```python
from build123d import *

# Parameters (mm, degrees)
SKETCH1_W                                 = 25.4
SKETCH1_H                                 = 50.8
SKETCH1_W_2                               = 20.32
SKETCH1_H_2                               = 45.72
VERSAFRAME_VERSAFRAME_2_X_1_X_0_1_1_DEPTH = 889
CUT_EXTRUDE1_DEPTH                        = 890.725418317
CUT_EXTRUDE1_DEPTH_BACK                   = 890.725418317
SKETCH2_R                                 = 14.2875
CUT_EXTRUDE2_DEPTH                        = 890.725418317
CUT_EXTRUDE2_DEPTH_BACK                   = 890.725418317
SKETCH3_R                                 = 2.07
SKETCH3_R_2                               = 3.175


with BuildPart() as part:
    # Sketch1 → Versaframe VERSAFRAME 2 X 1 X 0.1 (1) (new body)
    with BuildSketch(Plane(origin=(0, 0, 0), x_dir=(1, 0, 0), z_dir=(0, 1, 0))):
        Rectangle(SKETCH1_W, SKETCH1_H)
        Rectangle(SKETCH1_W_2, SKETCH1_H_2, mode=Mode.SUBTRACT)
    extrude(amount=VERSAFRAME_VERSAFRAME_2_X_1_X_0_1_1_DEPTH)

    # Sketch2 → Cut-Extrude1 (cut, two sides: drawn at the far end of the back side and taken through both)
    with BuildSketch(Plane(origin=(12.7, 0, 0), x_dir=(0, 0, -1), z_dir=(1, 0, 0)).offset(-CUT_EXTRUDE1_DEPTH_BACK)):
        with Locations((0, 31.75)):
            Circle(SKETCH2_R)
    extrude(amount=CUT_EXTRUDE1_DEPTH + CUT_EXTRUDE1_DEPTH_BACK, mode=Mode.SUBTRACT)

    # Sketch3 → Cut-Extrude2 (cut, two sides: drawn at the far end of the back side and taken through both)
    with BuildSketch(Plane(origin=(12.7, 0, 0), x_dir=(0, 0, -1), z_dir=(1, 0, 0)).offset(-CUT_EXTRUDE2_DEPTH_BACK)):
        with Locations((-12.7, 879.475)):
            Circle(SKETCH3_R)
        with Locations((-12.7, 860.425)):
            Circle(SKETCH3_R)
        with Locations((0, 869.95)):
            Circle(SKETCH3_R_2)
        with Locations((12.7, 860.425)):
            Circle(SKETCH3_R)
        with Locations((12.7, 879.475)):
            Circle(SKETCH3_R)
    extrude(amount=CUT_EXTRUDE2_DEPTH + CUT_EXTRUDE2_DEPTH_BACK, mode=Mode.SUBTRACT)


solid = part.part
```
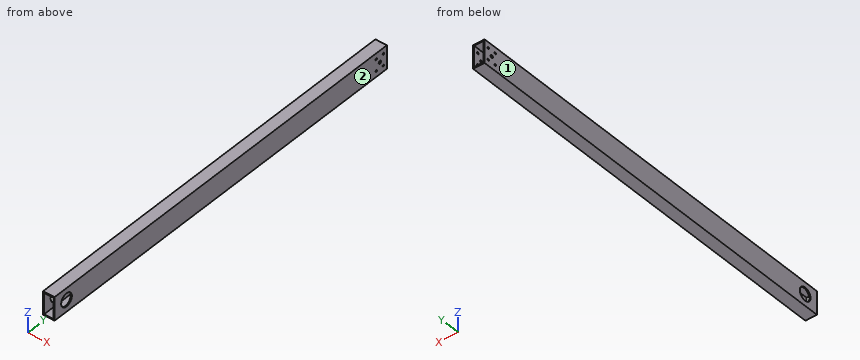
Work out the finished part from the listing and answer in its coordinate system (mm). Face numbers are marked on the shaded views. Give positions to 0.01 mm unless a question says otherwise; leave off trailing zeros. Write each loop counter-clockwise with the first axis right and the second up, starting at its lowest first coordinate (ties: lowest second). Pieces come first, ordered by that corner, then holes. Notation, with made-up numbers: (63.5, 14) - (106.5, 14) arc R26 ccw to (106.5, 35) - close; hole circle Ø9 at (21.25, 44.25). An arc over 180 degrees is marked (long way). Use one line per item in the form item = value.
1. A cutting plane is placed at B-B (y = 31.75). Write down the section's boundary in (x, z).
Filled in:
outline = (-12.7, -25.4) - (12.7, -25.4) - (12.7, -14.29) - (10.16, -14.29) - (10.16, -22.86) - (-10.16, -22.86) - (-10.16, -14.29) - (-12.7, -14.29) - close; (-12.7, 14.29) - (-10.16, 14.29) - (-10.16, 22.86) - (10.16, 22.86) - (10.16, 14.29) - (12.7, 14.29) - (12.7, 25.4) - (-12.7, 25.4) - close
2. Determine the mould class of the marked faces 1 and 2 for opening direction X: released by +X, released by -X, zero draft, split by the parting line, or undercut.
Filled in:
face_1 = released by -X
face_2 = released by +X
3. A cutting plane is placed at A-A (x = 5.5). Write down the section's boundary in (y, z).
Filled in:
outline = (0, -25.4) - (889, -25.4) - (889, -22.86) - (0, -22.86) - close; (0, 22.86) - (889, 22.86) - (889, 25.4) - (0, 25.4) - close
4. Consider L1, parallel to Z at x = -7.5, y = 272.5; L2, parallel to X at y = 582, z = 13; L3, parallel to Y at x = 11.05, z = -12.7 (3 decimals). Determine where each line is inside the solid, lowest interval first.
Filled in:
L1 = -25.4 to -22.86, 22.86 to 25.4
L2 = -12.7 to -10.16, 10.16 to 12.7
L3 = 0 to 25.205, 38.295 to 858.355, 862.495 to 877.405, 881.545 to 889
5. A cutting plane is placed at C-C (y = 812). Write down the section's boundary in (x, z), and give its area (3 significant figures).
Filled in:
outline = (-12.7, -25.4) - (12.7, -25.4) - (12.7, 25.4) - (-12.7, 25.4) - close; hole (-10.16, -22.86) - (10.16, -22.86) - (10.16, 22.86) - (-10.16, 22.86) - close
area = 361 mm^2
6. This flat-tipped pin is pushed along its axis until it touches: pin 1 Ø5.5 at (y, z) = (860.425, 12.7) entering from +X. Where does it stop, or does it pass through?
Filled in:
pin_1 = 12.7
